```python
from build123d import *

# Parameters (mm, degrees)
PAD013_DEPTH    = 7
PAD014_DEPTH    = 5
FILLET018_R     = 0.25
FILLET019_R     = 0.5
CHAMFER001_SIZE = 0.1


with BuildPart() as part:
    # Sketch035 → Pad013 (new body)
    with BuildSketch(Plane.XY):
        with BuildLine():
            Line((3.125, 3.095168), (-3.125, 3.095168))
            Line((-3.125, 3.095168), (-3.125, 0.745168))
            ThreePointArc((-3.125, 0.745168), (-3.79, 0), (-3.125, -0.745168))
            Line((-3.125, -1.945168), (-3.125, -0.745168))
            Line((-1.95, -3.204832), (-3.125, -1.945168))
            Line((1.95, -3.204832), (-1.95, -3.204832))
            Line((3.125, -1.945168), (1.95, -3.204832))
            Line((3.125, -0.745168), (3.125, -1.945168))
            ThreePointArc((3.125, -0.745168), (3.79, 0), (3.125, 0.745168))
            Line((3.125, 3.095168), (3.125, 0.745168))
        make_face()
    extrude(amount=PAD013_DEPTH)

    # Sketch036 (on Face12 of Pad013) → Pad014 (join)
    with BuildSketch(Plane.XY.offset(7)):
        Polygon((2, -1.154701), (2, 1.154701), (0, 2.309401), (-2, 1.154701), (-2, -1.154701), (0, -2.309401), align=None)
    extrude(amount=PAD014_DEPTH)

    # Fillet018
    fillet018_edges = [part.edges().sort_by_distance(p)[0] for p in [
        (1.95, -3.204832, 3.5),
        (3.125, -1.945168, 3.5),
        (-1.95, -3.204832, 3.5),
        (-3.125, -1.945168, 3.5),
        (-3.125, -0.745168, 3.5),
        (-3.125, 0.745168, 3.5),
        (-3.125, 3.095168, 3.5),
        (3.125, 3.095168, 3.5),
        (3.125, 0.745168, 3.5),
        (3.125, -0.745168, 3.5),
        (2, -1.154701, 9.5),
        (2, 1.154701, 9.5),
        (0, -2.309401, 9.5),
        (-2, -1.154701, 9.5),
        (-2, 1.154701, 9.5),
        (0, 2.309401, 9.5),
        (1, -1.732051, 7),
        (-1, -1.732051, 7),
        (-2, 0, 7),
        (-1, 1.732051, 7),
        (1, 1.732051, 7),
        (2, 0, 7),
    ]]
    fillet(fillet018_edges, radius=FILLET018_R)

    # Fillet019
    fillet019_edges = [part.edges().sort_by_distance(p)[0] for p in [
        (-1, -1.732051, 12),
        (0, -2.270726, 12),
        (1, -1.732051, 12),
        (1.966506, -1.135363, 12),
        (2, 0, 12),
        (1.966506, 1.135363, 12),
        (1, 1.732051, 12),
        (0, 2.270726, 12),
        (-1, 1.732051, 12),
        (-1.966506, 1.135363, 12),
        (-2, 0, 12),
        (-1.966506, -1.135363, 12),
    ]]
    fillet(fillet019_edges, radius=FILLET019_R)

    # Chamfer001
    chamfer001_edges = [part.edges().sort_by_distance(p)[0] for p in [
        (-3.125, 1.893693, 0),
        (-3.051777, 3.021944, 0),
        (0, 3.095168, 0),
        (3.051777, 3.021944, 0),
        (3.125, 1.893693, 0),
        (3.170748, 0.798061, 0),
        (3.79, 0, 0),
        (3.170748, -0.798061, 0),
        (3.125, -1.394444, 0),
        (3.107598, -1.938311, 0),
        (2.540973, -2.571277, 0),
        (1.940989, -3.184105, 0),
        (0, -3.204832, 0),
        (-1.940989, -3.184105, 0),
        (-2.540973, -2.571277, 0),
        (-3.107598, -1.938311, 0),
        (-3.125, -1.394444, 0),
        (-3.170748, -0.798061, 0),
        (-3.79, 0, 0),
        (-3.170748, 0.798061, 0),
    ]]
    chamfer(chamfer001_edges, length=CHAMFER001_SIZE)


solid = part.part
```
Geometry check sheet. Reference: the model listing, model coordinates, mm. A direction names the side the tool comes from. Give positions to 0.01 mm unless a question says otherwise; leave off trailing zeros. Write each loop counter-clockwise with the first axis right and the second up, starting at its lowest first coordinate (ties: lowest second). Pieces come first, ordered by that corner, then holes. Notation, with made-up numbers: (-27.5, 70.25) -> (22.5, 70.25) arc R18 ccw to (22.5, 93.25) -> close; hole circle Ø5 at (-22.75, 68.25). An arc over 180 degrees is marked (long way). Use one line per item in the form item = value.
Item 1: Scan lines: line 1 (Y direction, x = -0.75, z = 8.75); line 2 (Z direction, x = -3, y = 0); line 3 (X direction, y = 0, z = 10.25). Record each from-to range of solid material in increasing order.
Results list:
line_1 = -1.88 to 1.88
line_2 = 0 to 7
line_3 = -2 to 2
Item 2: Depth check by flat-ended pin: pin 1 Ø2 at (x, z) = (0, 10.5) entering from +Y; pin 2 Ø2 at (y, z) = (1.5, 4) entering from -X; pin 3 Ø2 at (y, z) = (-2.5, 10) entering from +X. Enter the tip coordinate at first touch or a pass-through.
Results list:
pin_1 = 2.27
pin_2 = -3.6
pin_3 = 1.4
Item 3: Sectioned sample at B-B on x = -2.5. Enter the section's corners in (y, z).
Results list:
outline = (-2.62, 0.1) -> (-2.47, 0) -> (3, 0) -> (3.1, 0.1) -> (3.1, 7) -> (-2.62, 7) -> close
Item 4: Sectioned sample at C-C on z = 6.75. Enter the section's corners in (x, y) (3 decimals).
Results list:
outline = (-3.291, -0.707) arc R0.25 cw to (-3.125, -0.942) -> (-3.125, -1.847) arc R0.25 ccw to (-3.058, -2.017) -> (-2.024, -3.125) arc R0.25 ccw to (-1.841, -3.205) -> (1.841, -3.205) arc R0.25 ccw to (2.024, -3.125) -> (3.058, -2.017) arc R0.25 ccw to (3.125, -1.847) -> (3.125, -0.942) arc R0.25 cw to (3.291, -0.707) arc R0.75 ccw to (3.291, 0.707) arc R0.25 cw to (3.125, 0.942) -> (3.125, 2.845) arc R0.25 ccw to (2.875, 3.095) -> (-2.875, 3.095) arc R0.25 ccw to (-3.125, 2.845) -> (-3.125, 0.942) arc R0.25 cw to (-3.291, 0.707) arc R0.75 ccw to start
Item 5: Sectioned sample at A-A on z = 10.5. Enter the section's corners in (x, y) (3 decimals), plus the area to 3 significant figures.
Results list:
outline = (-2, -1.01) arc R0.25 ccw to (-1.875, -1.227) -> (-0.125, -2.237) arc R0.25 ccw to (0.125, -2.237) -> (1.875, -1.227) arc R0.25 ccw to (2, -1.01) -> (2, 1.01) arc R0.25 ccw to (1.875, 1.227) -> (0.125, 2.237) arc R0.25 ccw to (-0.125, 2.237) -> (-1.875, 1.227) arc R0.25 ccw to (-2, 1.01) -> close
area = 13.8 mm2
Item 6: Access from +Z, -Z, +X, -X, +Y, -Y to the whole of each face (thin tool, end or side, straight path). Record for faces 1 (the flat face through (2, 0, 9)), 2 (the flat face through (-3.125, -1.4, 3.5)), 3 (the flat face through (3.125, 2, 4)), 4 (the flat face through (3.125, -1.4, 3.5)).
Results list:
face_1 = +Z, +X, +Y, -Y
face_2 = +Z, -Z, -X, -Y
face_3 = +Z, -Z, +X, +Y
face_4 = +Z, -Z, +X, -Y
